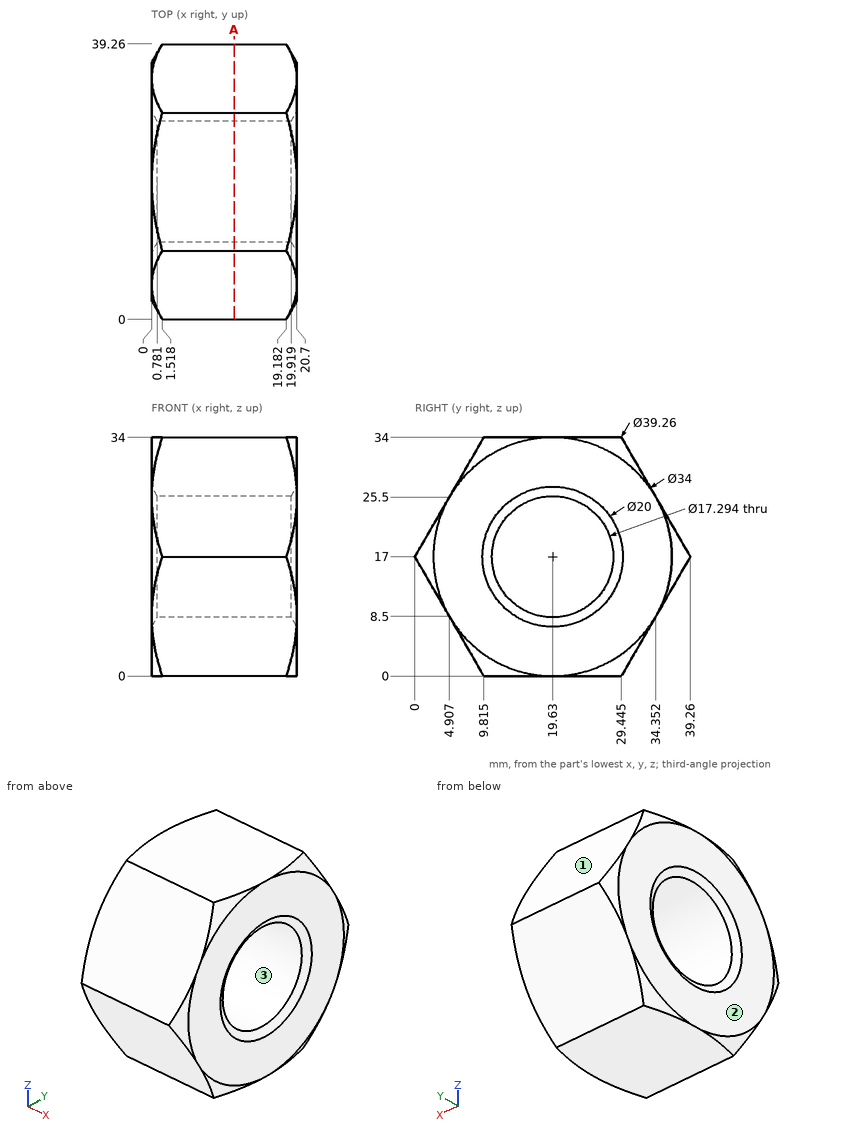
For this review, use the dimensioned drawing (mm, ordinates from the lowest corner) and the shaded views. Round coordinates to 2 decimals unless told otherwise and drop trailing zeros. Loops run counter-clockwise (first coordinate to the right, second up) from the corner with the lowest first, then second, coordinate; pieces in that order, holes last. Notation, with made-up numbers: M -26,-37.5 L -14,-37.5 A25 ccw -14,-9.5 Z; hole C 41,-0.5 d9. An arc over 180 degrees is marked long. Answer as a JSON object with one key per item and string values.
(1) Draft analysis for pull direction Z (two halves, no side actions). For the marked faces 1, 2 and 3, state which applies: released by +Z, released by -Z, zero draft, split by the parting line, or undercut.
Resolved:
{"face 1": "released by +Z", "face 2": "zero draft", "face 3": "undercut"}
(2) To check wall thickness, follow line 1 along Y through (x, z) = (15.25, 17) (1 decimal); line 2 along Z through (x, y) = (6.5, 16); line 3 along Z through (x, y) = (19.25, 26.5). State the ranges of each line that lie inside material, in increasing order.
Resolved:
{"line 1": "0 to 11, 28.3 to 39.3", "line 2": "0 to 9.15, 24.85 to 34", "line 3": "0 to 11.75, 22.25 to 34"}
(3) Take a section at A-A on x = 11.75. Give the boundary of the cut face in (y, z) (1 decimal).
Resolved:
{"outline": "M 0,17 L 9.8,0 L 29.4,0 L 39.3,17 L 29.4,34 L 9.8,34 Z; hole C 19.6,17 d17.3"}
(4) Clearance check with flat-ended pins moving along their axes: P1, Ø12, axis at x = 14.5, z = 29.5, coming from the +Y side; P2, Ø6, axis at x = 7.5, z = 16.5, coming from the +Y side; P3, Ø2, axis at x = 13, z = 29.5, coming from the +Y side. State where each tip first meets the part, or that it passes through.
Resolved:
{"P1": "y = 35.51", "P2": "y = 39.26", "P3": "y = 32.62"}
